Autodesk Inventor part; units mm, degrees
ref_plane "YZ Plane" through (0, 0, 0) normal (1, 0, 0) x (0, 1, 0)
ref_plane "XZ Plane" through (0, 0, 0) normal (0, 1, 0) x (-1, 0, 0)
ref_plane "XY Plane" through (0, 0, 0) normal (0, 0, 1) x (1, 0, 0)
sketch "Sketch1" plane through (0, 0, 0) normal (0, 1, 0) x (-1, 0, 0)
  line L0 (52.592, 0) -> (45.546, -26.296)
  line L1 (45.546, -26.296) -> (26.296, -45.546)
  line L2 (26.296, -45.546) -> (0, -52.592)
  line L3 (0, -52.592) -> (-26.296, -45.546)
  line L4 (-26.296, -45.546) -> (-45.546, -26.296)
  line L5 (-45.546, -26.296) -> (-52.592, 0)
  line L6 (-52.592, 0) -> (-45.546, 26.296)
  line L7 (-45.546, 26.296) -> (-26.296, 45.546)
  line L8 (-26.296, 45.546) -> (0, 52.592)
  line L9 (0, 52.592) -> (26.296, 45.546)
  line L10 (26.296, 45.546) -> (45.546, 26.296)
  line L11 (45.546, 26.296) -> (52.592, 0)
  point P0 (0, 0)
  point P1 (0, 0)
  dimension "d0" = 50.8
extrude "Extrusion1" add sketch "Sketch1" along normal blind 76.2
sketch "Sketch2" plane through (0, 76.2, 0) normal (0, 1, 0) x (1, 0, 0)
  line L0 (-48.1743, 0) -> (-41.7202, 24.0871)
  line L1 (-41.7202, 24.0871) -> (-24.0871, 41.7202)
  line L2 (-24.0871, 41.7202) -> (0, 48.1743)
  line L3 (0, 48.1743) -> (24.0871, 41.7202)
  line L4 (24.0871, 41.7202) -> (41.7202, 24.0871)
  line L5 (41.7202, 24.0871) -> (48.1743, 0)
  line L6 (48.1743, 0) -> (41.7202, -24.0871)
  line L7 (41.7202, -24.0871) -> (32.9037, -32.9037)
  line L8 (-32.9037, -32.9037) -> (-41.7202, -24.0871)
  line L9 (-41.7202, -24.0871) -> (-48.1743, 0)
  line L10 (-52.592, 0) -> (-45.546, -26.296)
  line L11 (-32.9037, -32.9037) -> (-32.9037, -66.8246)
  line L12 (-32.9037, -66.8246) -> (32.9037, -66.8246)
  line L13 (32.9037, -66.8246) -> (32.9037, -32.9037)
  point P0 (0, 0)
  point P1 (0, 0)
  dimension "d3" = 4.2672
extrude "Extrusion2" cut sketch "Sketch2" against normal blind 71.9328
fillet "Fillet1" radius 1.905 4 edges at (-32.9037, 40.2336, 38.9384) (-32.9037, 40.2336, 32.9037) (32.9037, 40.2336, 38.9384) (32.9037, 40.2336, 32.9037)
sketch "Sketch3" plane through (0, 4.2672, 0) normal (0, 1, 0) x (1, 0, 0)
  circle A0 centre (0, 0) radius 12.954
  dimension "d7" = 25.908
extrude "Extrusion3" add sketch "Sketch3" along normal blind 97.3328
fillet "Fillet2" radius 8.89 14 edges at (52.592, 38.1, 0) (45.546, 38.1, -26.296) (26.296, 38.1, -45.546) (0, 38.1, -52.592) (-26.296, 38.1, -45.546) (-45.546, 38.1, -26.296) (-52.592, 38.1, 0) (-48.1743, 40.2336, 0) (-41.7202, 40.2336, -24.0871) (-24.0871, 40.2336, -41.7202) (0, 40.2336, -48.1743) (24.0871, 40.2336, -41.7202) (41.7202, 40.2336, -24.0871) (48.1743, 40.2336, 0)
properties part number "holder-12"
Check sheet for the modelled part. Datum: model origin and axes. Units: mm. A direction names the side the tool comes from. Coordinates: 2 decimals unless noted, no trailing zeros. Write each loop counter-clockwise with the first axis right and the second up, starting at its lowest first coordinate (ties: lowest second). Pieces come first, ordered by that corner, then holes. Notation, with made-up numbers: (11.25, 26) - (15.25, 26) arc R17 cw to (15.25, 50) - close; hole circle Ø6 at (-32.75, 44.5). An arc over 180 degrees is marked (long way). One line per question, with ' | ' between items.
Item 1: Sectioned sample at B-B on x = -9.5. Record the boundary of the cut face in (y, z).
Determined:
outline: (0, -50.05) - (76.2, -50.05) - (76.2, -45.63) - (4.27, -45.63) - (4.27, -8.81) - (101.6, -8.81) - (101.6, 8.81) - (4.27, 8.81) - (4.27, 50.05) - (0, 50.05) - close
Item 2: Sectioned sample at C-C on y = 86. Record the boundary of the cut face in (x, z), plus the area to 3 significant figures.
Determined:
outline: circle Ø25.91 at (0, 0) | area: 527 mm2
Item 3: Gauge pin test, flat ends, axial feed: P1, Ø12, axis at x = -13, y = 48, coming from the +Z side; P2, Ø1.5, axis at x = -19, z = -24.5, coming from the -Y side; P3, Ø5, axis at y = 79.5, z = -23, coming from the +X side; P4, Ø2, axis at y = 74, z = -37, coming from the -X side. Record the tip position at first contact, or that the pin passes through.
Determined:
P1: stops at z = 10.9 | P2: stops at y = 0 | P3: passes through | P4: stops at x = -35.84
Item 4: Access from +Z, -Z, +X, -X, +Y, -Y to the whole of each face (thin tool, end or side, straight path). Record for faces 5 (the face through (37.65, 40.74, 28.16)), 6 (the face through (-34.051, 39.73, 36.087)), 7 (the face through (48.806, 37.567, 14.13)).
Determined:
face 5: +Y | face 6: +Z, +Y | face 7: +Z, +X, +Y, -Y
Item 5: Sectioned sample at A-A on z = 0. Record the boundary of the cut face in (x, y), plus the area to 3 significant figures.
Determined:
outline: (-52.28, 0) - (52.28, 0) - (52.28, 76.2) - (47.86, 76.2) - (47.86, 4.27) - (12.95, 4.27) - (12.95, 101.6) - (-12.95, 101.6) - (-12.95, 4.27) - (-47.86, 4.27) - (-47.86, 76.2) - (-52.28, 76.2) - close | area: 3,600 mm2
Item 6: Sectioned sample at D-D on z = -11.5. Record the boundary of the cut face in (x, y), plus the area to 3 significant figures.
Determined:
outline: (-49.51, 0) - (49.51, 0) - (49.51, 76.2) - (45.09, 76.2) - (45.09, 4.27) - (5.96, 4.27) - (5.96, 101.6) - (-5.96, 101.6) - (-5.96, 4.27) - (-45.09, 4.27) - (-45.09, 76.2) - (-49.51, 76.2) - close | area: 2,220 mm2
Item 7: Thickness scan on line 1 (X direction, y = 49.5, z = 5.5); line 2 (X direction, y = 36, z = 5); line 3 (Y direction, x = 16.5, z = 45). Record the ranges inside material, lowest first. Write a range as [from, to].
Determined:
line 1: x = [-51.12, -46.7], [-11.73, 11.73], [46.7, 51.12] | line 2: x = [-51.25, -46.83], [-11.95, 11.95], [46.83, 51.25] | line 3: y = [0, 4.27]
Item 8: Mould release check, pull along X, two halves, no side actions. Record for faces 1 (the face through (-37.533, 40.737, 28.274)), 2 (the face through (26.167, 38.633, -45.258)), 3 (the face through (-23.96, 39.73, -41.43)), 4 (the face through (-52.28, 38.63, -0.03)): pulls with the +X half, pulls with the -X half, needs draft (parallel to the pull), parting line crosses it, or undercut.
Determined:
face 1: undercut | face 2: pulls with the +X half | face 3: undercut | face 4: pulls with the -X half
